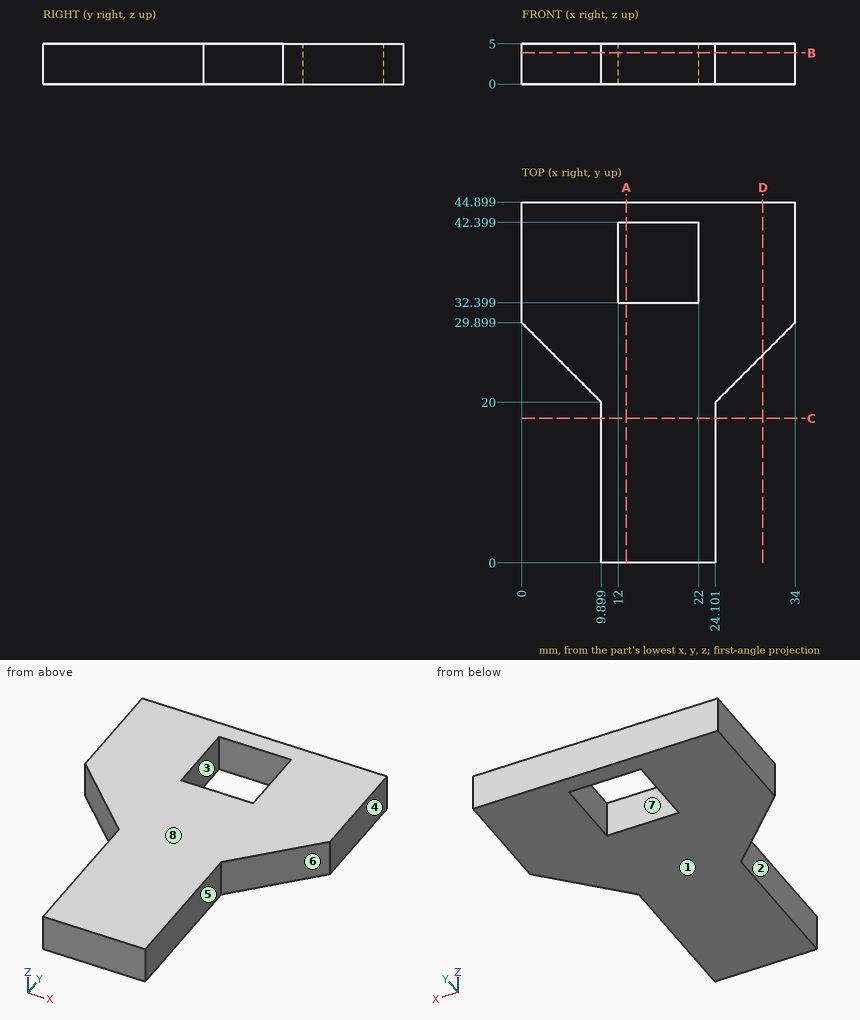
Can you work these out from the drawing? Everything is in mm from the part's minimum corner. A direction names the side the tool comes from. Give positions to 0.01 mm unless a question says otherwise; leave off trailing zeros. Order: outer loops, then holes, each group sorted by start corner. A loop starts at its lowest first (then second) coordinate and runs counter-clockwise, first axis right, second up. Notation, with made-up numbers: M -13.75,75.25 L 19.25,75.25 A11 ccw 19.25,89.25 Z; hole C 31,43.5 d4. An arc over 180 degrees is marked long. Use a Markdown table: item, result. Add a question column.
Item 1: For the marked faces 1, 2, 3, 4 and 5, which set-ups out of +Z, -Z, +X, -X, +Y, -Y let a thin tool reach every point of the face, with its end or its side?
Item 2: Suppose I cut it at A-A (x = 13). List the corners of the cut face in (y, z) for me.
Item 3: Suppose I cut it at D-D (x = 30). List the corners of the cut face in (y, z) for me, then the cut area to 3 significant figures.
Item 4: We'd pull the mould along Y, two halves only. Please class the marked faces 6, 7 and 8: +Y half, -Y half, draft (parallel to the pull), parting line (faces both ways), or undercut.
Item 5: Suppose I cut it at B-B (z = 3.9). List the corners of the cut face in (x, y) for me.
Item 6: Suppose I cut it at C-C (y = 18). List the corners of the cut face in (x, z) for me.
Item 7: If I drill on L1, parallel to Y at x = 14.5, z = 2.8; L2, parallel to X at y = 37, z = 1.85; L3, parallel to X at y = 2, z = 3.8, over which ranges is the centre line in solid material (lowest first)? Write a range as [from, to].
Item 8: Will these pins go through, and if not, where does the flat tip stop? pin 1 (1.5 mm diameter, centred on x = 16.5, z = 1.5, fed in from -Y); pin 2 (1 mm diameter, centred on y = 18.5, z = 1.5, fed in from +X); pin 3 (2.5 mm diameter, centred on y = 9.5, z = 2.5, fed in from -X).
Answer sheet:
| question | item | result |
|---|---|---|
| 1 | face 1 | -Z, +X, -X, +Y, -Y |
| 1 | face 2 | +Z, -Z, -X, -Y |
| 1 | face 3 | +Z, -Z |
| 1 | face 4 | +Z, -Z, +X, +Y, -Y |
| 1 | face 5 | +Z, -Z, +X, -Y |
| 2 | outline | M 0,0 L 32.4,0 L 32.4,5 L 0,5 Z; M 42.4,0 L 44.9,0 L 44.9,5 L 42.4,5 Z |
| 3 | outline | M 25.9,0 L 44.9,0 L 44.9,5 L 25.9,5 Z |
| 3 | area | 95.0 mm² |
| 4 | face 6 | -Y half |
| 4 | face 7 | undercut |
| 4 | face 8 | draft |
| 5 | outline | M 0,29.9 L 9.9,20 L 9.9,0 L 24.1,0 L 24.1,20 L 34,29.9 L 34,44.9 L 0,44.9 Z; hole M 12,32.4 L 22,32.4 L 22,42.4 L 12,42.4 Z |
| 6 | outline | M 9.9,0 L 24.1,0 L 24.1,5 L 9.9,5 Z |
| 7 | L1 | y = [0, 32.4], [42.4, 44.9] |
| 7 | L2 | x = [0, 12], [22, 34] |
| 7 | L3 | x = [9.9, 24.1] |
| 8 | pin 1 | stops at y = 0 |
| 8 | pin 2 | stops at x = 24.1 |
| 8 | pin 3 | stops at x = 9.9 |
